Geometry: final body of the model. Coordinates: model frame, mm. Give positions to 0.01 mm unless a question says otherwise; leave off trailing zeros. Loops run counter-clockwise (first coordinate to the right, second up) from the corner with the lowest first, then second, coordinate; pieces in that order, holes last. Notation, with made-up numbers: (11.5, 34.5) -> (16.5, 34.5) arc R32 ccw to (16.5, 65.5) -> close; hole circle Ø4 at (63.5, 24.25). An arc over 180 degrees is marked (long way). Answer in a Markdown table with one row per item. Add a question column.
from build123d import *

# Parameters (mm, degrees)
F0_W     = 228.6
F0_H     = 63.5
F1_DEPTH = 38.1
F2_R     = 3.175
F3_DEPTH = 25.4


with BuildPart() as f1:
    # F0 (on Top) → F1 (new body)
    with BuildSketch(Plane.XY):
        Rectangle(F0_W, F0_H)
    extrude(amount=F1_DEPTH)

    # F2 (on face) → F3 (cut)
    with BuildSketch(Plane.XY.offset(38.1)):
        with Locations((-88.9, -12.7)):
            Circle(F2_R)
        with Locations((-88.9, 12.7)):
            Circle(F2_R)
        with Locations((-63.5, -12.7)):
            Circle(F2_R)
        with Locations((-63.5, 12.7)):
            Circle(F2_R)
        with Locations((-38.1, -12.7)):
            Circle(F2_R)
        with Locations((-38.1, 12.7)):
            Circle(F2_R)
        with Locations((-12.7, -12.7)):
            Circle(F2_R)
        with Locations((-12.7, 12.7)):
            Circle(F2_R)
        with Locations((12.7, -12.7)):
            Circle(F2_R)
        with Locations((12.7, 12.7)):
            Circle(F2_R)
        with Locations((38.1, -12.7)):
            Circle(F2_R)
        with Locations((38.1, 12.7)):
            Circle(F2_R)
        with Locations((63.5, -12.7)):
            Circle(F2_R)
        with Locations((63.5, 12.7)):
            Circle(F2_R)
        with Locations((88.9, -12.7)):
            Circle(F2_R)
        with Locations((88.9, 12.7)):
            Circle(F2_R)
    extrude(amount=-F3_DEPTH, mode=Mode.SUBTRACT)


solid = f1.part
(1) Cut plane B-B on x = -12.7. Return the cut outline in (y, z) (3 decimals).
(2) Cut plane A-A on z = 25. State how many separate pieces and enclosed holes the cut face has, then the cut area to 3 significant figures.
(3) Pin query (flat end, axial travel): pin 1 Ø3 at (x, y) = (-64.5, -13) entering from +Z. Return the tip coordinate at first contact, or that it passes through.
(4) Draft query along Y for faces 1 (the flat face through (13, -13, 12.7)), 2 (the flat face through (-2, 0, 0)), 3 (the flat face through (-2, 31.75, 19)). Return one class per face: +Y half, -Y half, draft (parallel to the pull), parting line (faces both ways), or undercut.
(5) Material intervals for line 1 along Y through (x, z) = (63.5, 26.25) (3 decimals); line 2 along Y through (x, z) = (90, 16.5); line 3 along Z through (x, y) = (90, 13.5), sorted ascending. Write a range as from..to.
Answer list:
| question | item | result |
|---|---|---|
| 1 | outline | (-31.75, 0) -> (31.75, 0) -> (31.75, 38.1) -> (15.875, 38.1) -> (15.875, 12.7) -> (9.525, 12.7) -> (9.525, 38.1) -> (-9.525, 38.1) -> (-9.525, 12.7) -> (-15.875, 12.7) -> (-15.875, 38.1) -> (-31.75, 38.1) -> close |
| 2 | separate pieces | 1 |
| 2 | enclosed holes | 16 |
| 2 | area | 14,000 mm² |
| 3 | pin 1 | stops at z = 12.7 |
| 4 | face 1 | undercut |
| 4 | face 2 | draft |
| 4 | face 3 | +Y half |
| 5 | line 1 | y = -31.75..-15.875, -9.525..9.525, 15.875..31.75 |
| 5 | line 2 | y = -31.75..-15.68, -9.72..9.72, 15.68..31.75 |
| 5 | line 3 | z = 0..12.7 |
